Check sheet for the modelled part. Datum: model origin and axes. Units: mm. Face numbers are marked on the shaded views. A direction names the side the tool comes from. Round coordinates to 2 decimals unless told otherwise and drop trailing zeros. Loops run counter-clockwise (first coordinate to the right, second up) from the corner with the lowest first, then second, coordinate; pieces in that order, holes last. Notation, with made-up numbers: M 65,73.5 L 82,73.5 A29 ccw 82,106.5 Z; hole C -25.75,69.25 d9. An arc over 180 degrees is marked long. One line per question, with ' | ' between items. Start each with the question number.
(1) Section check C-C (z = 15). Record the boundary of the cut face in (x, y), and give its area (3 significant figures).
(2) Draft check along Z on the marked faces 1, 2 and 3. Enter one of: +Z half, -Z half, draft (parallel to the pull), parting line (faces both ways), or undercut.
(3) Tool access check on the marked faces 4, 5 and 6. Record the directions out of +Z, -Z, +X, -X, +Y, -Y that give a thin tool (end or side, any length) a straight path to the whole face; none if there is none.
(4) Section check A-A (x = -40). Record the boundary of the cut face in (y, z).
(5) Section check D-D (z = 0). Record the boundary of the cut face in (x, y), and give its area (3 significant figures).
(6) Go/stop test with flat-tipped pins: P1, Ø5, axis at x = 1, y = 12.5, coming from the +Z side; P2, Ø3, axis at y = 11.5, z = 1.5, coming from the -X side; P3, Ø6.5, axis at x = -38.5, z = 14.5, coming from the +Y side. Record where each tip stops, or that it passes through.
(7) Thickness scan on probe 1 along Z at (x, y) = (40, 12.75); probe 2 along X at (y, z) = (8.5, -15); probe 3 along Z at (x, y) = (-39.5, 11). Record the ranges inside material, lowest first. Write a range as [from, to].
(8) Section check B-B (y = 6.25). Record the boundary of the cut face in (x, z), and give its area (3 significant figures).
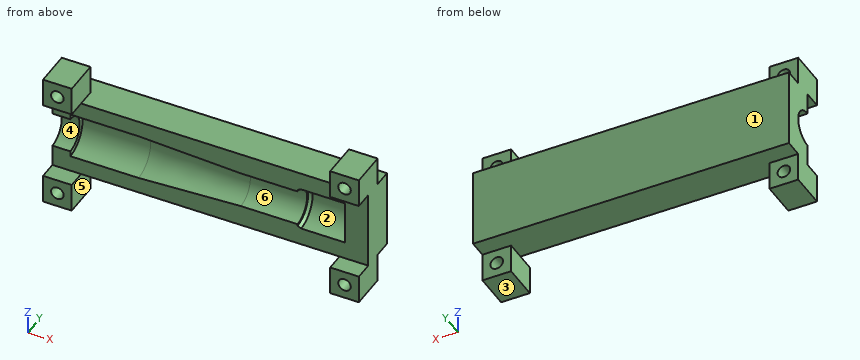
Autodesk Inventor part; units mm, degrees
ref_plane "YZ Plane" through (0, 0, 0) normal (1, 0, 0) x (0, 1, 0)
ref_plane "XZ Plane" through (0, 0, 0) normal (0, 1, 0) x (-1, 0, 0)
ref_plane "XY Plane" through (0, 0, 0) normal (0, 0, 1) x (1, 0, 0)
sketch "Sketch1" plane through (0, 0, 0) normal (0, 1, 0) x (-1, 0, 0)
  line L0 (44, 11) -> (-44, 11)
  line L1 (-44, 11) -> (-44, -11)
  line L2 (-44, -11) -> (44, -11)
  line L3 (44, -11) -> (44, 11)
  line L4 (44, 11) -> (-44, -11) construction
  line L5 (-44, 11) -> (44, -11) construction
  line L6 (36, 19) -> (44, 19)
  line L7 (44, 19) -> (44, 11)
  line L8 (44, 11) -> (36, 11)
  line L9 (36, 11) -> (36, 19)
  line L10 (36, 19) -> (44, 11) construction
  line L11 (44, 19) -> (36, 11) construction
  line L12 (36, -19) -> (44, -19)
  line L13 (44, -19) -> (44, -11)
  line L14 (44, -11) -> (36, -11)
  line L15 (36, -11) -> (36, -19)
  line L16 (36, -19) -> (44, -11) construction
  line L17 (44, -19) -> (36, -11) construction
  line L18 (-36, 19) -> (-44, 19)
  line L19 (-44, 19) -> (-44, 11)
  line L20 (-44, 11) -> (-36, 11)
  line L21 (-36, 11) -> (-36, 19)
  line L22 (-36, 19) -> (-44, 11) construction
  line L23 (-44, 19) -> (-36, 11) construction
  line L24 (-36, -19) -> (-44, -19)
  line L25 (-44, -19) -> (-44, -11)
  line L26 (-44, -11) -> (-36, -11)
  line L27 (-36, -11) -> (-36, -19)
  line L28 (-36, -19) -> (-44, -11) construction
  line L29 (-44, -19) -> (-36, -11) construction
  circle A0 centre (40, 15) radius 1.75
  circle A1 centre (40, -15) radius 1.75
  circle A2 centre (-40, 15) radius 1.75
  circle A3 centre (-40, -15) radius 1.75
  point P0 (0, 0)
  dimension "d0" = 22
  dimension "d1" = 88
  dimension "d2" = 8
  dimension "d3" = 8
  dimension "d8" = 3.5
  dimension "d9" = 3.5
  dimension "d10" = 3.5
  dimension "d11" = 3.5
  dimension "d24" = 30
  dimension "d25" = 80
extrude "Extrusion1" add sketch "Sketch1" along normal blind 10 contours L3 L2 L1 L0
extrude "Extrusion2" add sketch "Sketch1" along normal blind 5 contours L0 L9 L6 L7 | L13 L12 L15 L2 | L0 L19 L18 L21 | L27 L24 L25 L2
sketch "Sketch3" plane through (0, 10, 0) normal (0, 1, 0) x (1, 0, 0)
  line L0 (44, 11) -> (44, 19)
  line L1 (-44, -11) -> (44, -11)
  line L2 (44, -11) -> (44, 11)
  line L3 (44, 11) -> (-44, 11)
  line L4 (-44, 11) -> (-44, -11)
  line L5 (-44, -11) -> (44, 11) construction
  line L6 (44, -11) -> (-44, 11) construction
  line L7 (-36, -19) -> (-36, -11)
  line L8 (-44, -11) -> (-36, -11)
  line L9 (-44, -11) -> (-44, -19)
  line L10 (-44, -19) -> (-36, -19)
  circle A0 centre (-40, -15) radius 1.75
  line L11 (-36, 11) -> (-44, 11)
  line L12 (-36, 11) -> (-36, 19)
  line L13 (-36, 19) -> (-44, 19)
  line L14 (-44, 19) -> (-44, 11)
  circle A1 centre (-40, 15) radius 1.75
  line L15 (36, 19) -> (36, 11)
  line L16 (44, 11) -> (36, 11)
  line L17 (44, 11) -> (44, 19)
  line L18 (44, 19) -> (36, 19)
  circle A2 centre (40, 15) radius 1.75
  line L19 (36, -11) -> (44, -11)
  line L20 (36, -11) -> (36, -19)
  line L21 (36, -19) -> (44, -19)
  line L22 (44, -19) -> (44, -11)
  circle A3 centre (40, -15) radius 1.75
  point P0 (0, 0)
extrude "Extrusion3" add sketch "Sketch3" along normal blind 10 contours L2 L1 L4 L3
extrude "Extrusion4" add sketch "Sketch3" along normal mid plane 10 contours L3 L15 L18 L0 | L22 L21 L20 L1 | L3 L14 L13 L12 | L7 L10 L9 L1
sketch "Sketch2" plane through (0, 10, 0) normal (0, 1, 0) x (1, 0, 0)
  line L0 (-98.02, 0) -> (97.5, 0)
  line L1 (-39, 5) -> (-39, 6.5)
  line L2 (-39, 6.5) -> (-20, 6.5)
  line L3 (-20, 6.5) -> (8.5, 5.1)
  line L4 (8.5, 5.1) -> (24.3, 5.1)
  line L5 (24.3, 5.1) -> (24.3, 5.6)
  line L6 (24.3, 5.6) -> (25.3, 6.1)
  line L7 (25.3, 6.1) -> (37.5, 6.1)
  line L8 (37.5, 6.1) -> (37.5, 0)
  line L9 (-38.5, 0) -> (37.5, 0)
  line L10 (-44, 11) -> (-44, -11)
  line L11 (-39, 5) -> (-44, 5)
  line L12 (-44, 5) -> (-44, 0)
  point P0 (0, 0)
  dimension "d12" = 13
  dimension "d13" = 12.2
  dimension "d14" = 1
  dimension "d15" = 0.5
  dimension "d16" = 10.2
  dimension "d17" = 76.5
  dimension "d18" = 13.2
  dimension "d19" = 19
  dimension "d20" = 5
  dimension "d21" = 29
  dimension "d23" = 10
revolve "Revolution1" cut sketch "Sketch2" angle 360 about axis through (-98.02, 10, 0) along (1, 0, 0)
extrude "Extrusion6" cut sketch "Sketch1" along normal blind 10 contours L3 L2 L1 L0
extrude "Extrusion7" cut sketch "Sketch1" along normal blind 5 contours L3 L2 L1 L0 | L0 L9 L6 L7 | L13 L12 L15 L2 | L0 L19 L18 L21 | L27 L24 L25 L2 | A1 | A2
equation "\"d9\" = d8"
equation "\"d10\" = d8"
equation "\"d11\" = d8"
properties part number "stick_antenna__case_cap"
The answers:
1) outline: M -44,5 L -41.75,5 L -41.75,15 L -44,15 Z; M -38.25,5 L -36,5 L -36,15 L -38.25,15 Z; M 36,5 L 38.25,5 L 38.25,15 L 36,15 Z; M 41.75,5 L 44,5 L 44,15 L 41.75,15 Z | area: 90.0 mm²
2) face 1: draft | face 2: undercut | face 3: -Z half
3) face 4: -X, -Y | face 5: -Z, +Y, -Y | face 6: -Y
4) outline: M 5,-19 L 15,-19 L 15,-16.75 L 5,-16.75 Z; M 5,-13.25 L 15,-13.25 L 15,-11 L 20,-11 L 20,11 L 15,11 L 15,13.25 L 5,13.25 L 5,11 L 10,11 L 10,5 A5 cw 10,-5 L 10,-11 L 5,-11 Z; M 5,16.75 L 15,16.75 L 15,19 L 5,19 Z
5) outline: M -44,15 L -39,15 L -39,16.5 L -20,16.5 L 8.5,15.1 L 24.3,15.1 L 24.3,15.6 L 25.3,16.1 L 37.5,16.1 L 37.5,10 L 44,10 L 44,20 L -44,20 Z | area: 405 mm²
6) P1: z = 11 | P2: x = 37.5 | P3: y = 15
7) probe 1: [-19, -16.75], [-13.25, 13.25], [16.75, 19] | probe 2: [-44, -41.75], [-38.25, -36], [36, 38.25], [41.75, 44] | probe 3: [-19, -16.68], [-13.32, -4.9], [4.9, 13.32], [16.68, 19]
8) outline: M -44,-19 L -36,-19 L -36,-11 L -44,-11 Z; M -44,11 L -36,11 L -36,19 L -44,19 Z; M 36,-19 L 44,-19 L 44,-11 L 36,-11 Z; M 36,11 L 44,11 L 44,19 L 36,19 Z; hole C -40,-15 d3.5; hole C -40,15 d3.5; hole C 40,-15 d3.5; hole C 40,15 d3.5 | area: 218 mm²
